from build123d import *

# Parameters (mm, degrees)
BOSS_EXTRUDE1_DEPTH     = 392
CUT_EXTRUDE1_DEPTH      = 395.732071568
CUT_EXTRUDE1_DEPTH_BACK = 395.732071568
SKETCH2_W               = 4
SKETCH2_H               = 36
SKETCH3_R               = 7
CUT_EXTRUDE2_DEPTH      = 10


with BuildPart() as part:
    # Sketch1 → Boss-Extrude1 (new body)
    with BuildSketch(Plane(origin=(0, 0, 0), x_dir=(1, 0, 0), z_dir=(0, 1, 0))):
        with BuildLine():
            Line((-27.499872145, 29.213153277), (-67.499872145, 29.213153277))
            Line((-67.499872145, 29.213153277), (-67.499872145, -10.786846723))
            Line((-67.499872145, -10.786846723), (-66.499872145, -10.786846723))
            ThreePointArc((-66.499872145, -10.786846723), (-64.378551801, -9.908167067), (-63.499872145, -7.786846723))
            Line((-63.499872145, -7.786846723), (-63.499872145, 22.213153277))
            ThreePointArc((-63.499872145, 22.213153277), (-62.621192489, 24.334473621), (-60.499872145, 25.213153277))
            Line((-60.499872145, 25.213153277), (-30.499872145, 25.213153277))
            ThreePointArc((-30.499872145, 25.213153277), (-28.378551801, 26.091832933), (-27.499872145, 28.213153277))
            Line((-27.499872145, 28.213153277), (-27.499872145, 29.213153277))
        make_face()
    extrude(amount=BOSS_EXTRUDE1_DEPTH)

    # Sketch2 → Cut-Extrude1 (cut, two sides: drawn at the far end of the back side and taken through both)
    with BuildSketch(Plane(origin=(-63.499872145, 0, 0), x_dir=(0, 0, -1), z_dir=(1, 0, 0)).offset(-CUT_EXTRUDE1_DEPTH_BACK)):
        with Locations((27.213153277, 374)):
            Rectangle(SKETCH2_W, SKETCH2_H)
        with Locations((27.213153277, 18)):
            Rectangle(SKETCH2_W, SKETCH2_H)
    extrude(amount=CUT_EXTRUDE1_DEPTH + CUT_EXTRUDE1_DEPTH_BACK, mode=Mode.SUBTRACT)

    # Sketch3 → Cut-Extrude2 (cut)
    with BuildSketch(Plane(origin=(-63.499872145, 0, 0), x_dir=(0, 0, -1), z_dir=(1, 0, 0))):
        with Locations((9.213153277, 196)):
            Circle(SKETCH3_R)
        with Locations((9.213153277, 46)):
            Circle(SKETCH3_R)
        with Locations((9.213153277, 346)):
            Circle(SKETCH3_R)
    extrude(amount=-CUT_EXTRUDE2_DEPTH, mode=Mode.SUBTRACT)


solid = part.part
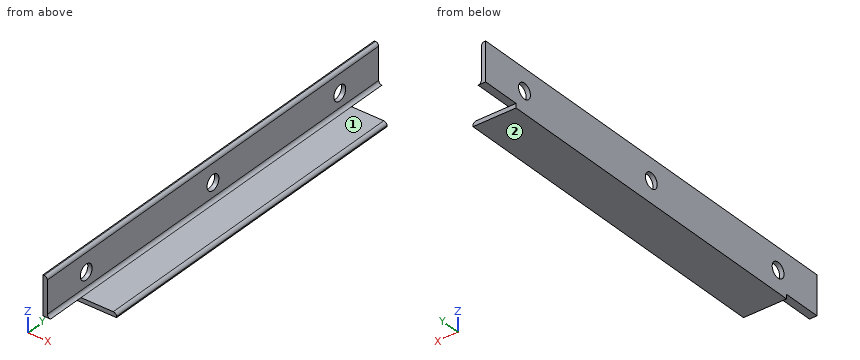
Can you work these out from the model? Positions are in its coordinate system, mm. Face numbers are marked on the shaded views. A direction names the side the tool comes from. Give positions to 0.01 mm unless a question says otherwise; leave off trailing zeros. Order: outer loops, then holes, each group sorted by start corner. A loop starts at its lowest first (then second) coordinate and runs counter-clockwise, first axis right, second up. Notation, with made-up numbers: M 31.5,5.25 L 70.5,5.25 A19 ccw 70.5,26.25 Z; hole C 30,-32 d8. An arc over 180 degrees is marked long. Use one line per item in the form item = value. Start each with the question number.
Item 1: If we section it at B-B (z = -5.5): Write out the boundary of the cut face in (x, y), then the cut area to 3 significant figures.
Item 2: Will these pins go through, and if not, where does the flat tip stop? pin 1 Ø10 at (y, z) = (168, -4) entering from +X; pin 2 Ø2 at (x, y) = (-64.5, 10.5) entering from -Z; pin 3 Ø2 at (x, y) = (-32.5, 247.5) entering from +Z.
Item 3: If we section it at D-D (x = -38): Write out the boundary of the cut face in (y, z), then the cut area to 3 significant figures.
Item 4: For the marked faces 1 and 2, which set-ups out of +Z, -Z, +X, -X, +Y, -Y let a thin tool reach every point of the face, with its end or its side?
Item 5: If we section it at A-A (y = 46): Write out the boundary of the cut face in (x, z), then the cut area to 3 significant figures.
Item 6: If we section it at C-C (y = 333.5): Write out the boundary of the cut face in (x, z), then the cut area to 3 significant figures.
Item 7: If I drill on line 1 along Y through (x, z) = (-55, -26); line 2 along X through (y, z) = (169, -16); line 3 along Z through (x, y) = (-58.5, 71), over which ranges is the centre line in solid material (lowest first)?
Outcome:
q1.outline = M -67.5,0 L -63.5,0 L -63.5,40.07 L -67.5,40.07 Z; M -67.5,51.93 L -63.5,51.93 L -63.5,190.07 L -67.5,190.07 Z; M -67.5,201.93 L -63.5,201.93 L -63.5,340.07 L -67.5,340.07 Z; M -67.5,351.93 L -63.5,351.93 L -63.5,392 L -67.5,392 Z
q1.area = 1,430 mm2
q2.pin_1 = -63.5
q2.pin_2 = -25.21
q2.pin_3 = -25.21
q3.outline = M 36,-29.21 L 356,-29.21 L 356,-25.21 L 36,-25.21 Z
q3.area = 1,280 mm2
q4.face_1 = +Z, +X, +Y, -Y
q4.face_2 = -Z, +X, -X, +Y, -Y
q5.outline = M -67.5,-29.21 L -27.5,-29.21 L -27.5,-28.21 A3 ccw -30.5,-25.21 L -60.5,-25.21 A3 cw -63.5,-22.21 L -63.5,-16.21 L -67.5,-16.21 Z; M -67.5,-2.21 L -63.5,-2.21 L -63.5,7.79 A3 ccw -66.5,10.79 L -67.5,10.79 Z
q5.area = 246 mm2
q6.outline = M -67.5,-29.21 L -27.5,-29.21 L -27.5,-28.21 A3 ccw -30.5,-25.21 L -60.5,-25.21 A3 cw -63.5,-22.21 L -63.5,7.79 A3 ccw -66.5,10.79 L -67.5,10.79 Z
q6.area = 302 mm2
q7.line_1 = 36 to 356
q7.line_2 = -67.5 to -63.5
q7.line_3 = -29.21 to -25.21
